```python
from build123d import *

# Parameters (mm, degrees)
SKETCH1_R                = 1.5
BOSS_EXTRUDE1_DEPTH      = 4
SKETCH2_W                = 10
SKETCH2_H                = 6
BOSS_EXTRUDE2_DEPTH      = 5
SKETCH7_W                = 6
SKETCH7_H                = 5
BOSS_EXTRUDE5_DEPTH      = 10
SKETCH4_R                = 2.5
BOSS_EXTRUDE3_DEPTH      = 10
BOSS_EXTRUDE3_DEPTH_BACK = 5


with BuildPart() as part:
    # Sketch1 → Boss-Extrude1 (new body)
    with BuildSketch(Plane.XY):
        Polygon((0, 0), (0, 30), (7.5, 30), (7.5, 0), (7.5, -2), (0, -2), align=None)
        with Locations((3.75, 26.5)):
            Circle(SKETCH1_R, mode=Mode.SUBTRACT)
        with Locations((3.75, 3.5)):
            Circle(SKETCH1_R, mode=Mode.SUBTRACT)
    extrude(amount=BOSS_EXTRUDE1_DEPTH)

    # Sketch2 → Boss-Extrude2 (add)
    with BuildSketch(Plane.XZ.offset(2)):
        with Locations((3.75, 3)):
            Rectangle(SKETCH2_W, SKETCH2_H)
    extrude(amount=BOSS_EXTRUDE2_DEPTH)

    # Sketch7 → Boss-Extrude5 (add)
    with BuildSketch(Plane.ZY.offset(1.25)):
        with Locations((3, -4.5)):
            Rectangle(SKETCH7_W, SKETCH7_H)
    extrude(amount=BOSS_EXTRUDE5_DEPTH)

    # Sketch4 → Boss-Extrude3 (add, two sides)
    with BuildSketch(Plane.XZ.offset(7)) as boss_extrude3_sk:
        with Locations((8.75, 3.5)):
            Circle(SKETCH4_R)
        with Locations((-11.25, 1.044308782)):
            Circle(SKETCH4_R)
    extrude(amount=BOSS_EXTRUDE3_DEPTH)
    extrude(boss_extrude3_sk.sketch, amount=-BOSS_EXTRUDE3_DEPTH_BACK)


solid = part.part
```
Could you check a few things on this model? Use its own coordinates, in mm. A direction names the side the tool comes from. Give positions to 0.01 mm unless a question says otherwise; leave off trailing zeros. Write each loop counter-clockwise with the first axis right and the second up, starting at its lowest first coordinate (ties: lowest second). Pieces come first, ordered by that corner, then holes. Notation, with made-up numbers: (34.25, 32.5) -> (57.25, 32.5) arc R22 ccw to (57.25, 69.5) -> close; hole circle Ø5 at (49.5, 2.5). An arc over 180 degrees is marked (long way). Write each question's results on one line, items separated by ' | '.
1. I want a section at B-B, the plane x = 3.75. Write out the boundary of the cut face in (y, z), then the cut area to 3 significant figures.
Check sheet entries:
outline: (-7, 0) -> (2, 0) -> (2, 4) -> (-2, 4) -> (-2, 6) -> (-7, 6) -> close; (5, 0) -> (25, 0) -> (25, 4) -> (5, 4) -> close; (28, 0) -> (30, 0) -> (30, 4) -> (28, 4) -> close | area: 134 mm²
2. I want a section at D-D, the plane x = -7.75. Write out the boundary of the cut face in (y, z).
Check sheet entries:
outline: (-7, 0) -> (-2, 0) -> (-2, 6) -> (-7, 6) -> close
3. If we mould it in two halves opening along X, with no side actions, what happens to faces 1 (the cylindrical face through (5.136, 2.925, 1.972)), 2 (the flat face through (9, -17, 4)), 3 (the flat face through (8.75, -4.5, 0.5))? For each: released by +X, released by -X, zero draft, split by the parting line, or undercut.
Check sheet entries:
face 1: undercut | face 2: zero draft | face 3: released by +X
4. On a 3-axis mill with a long thin cutter (end or side, diameter ignored), from which of +Z, -Z, +X, -X, +Y, -Y can I reach the whole of each face in a straight line? I mean faces 4 (the flat face through (0, 14, 2)), 5 (the flat face through (7.5, 14, 2)), 6 (the flat face through (2, 7, 0)), 7 (the flat face through (4, 14, 4)). Say none if no direction works.
Check sheet entries:
face 4: +Z, -Z, -X, +Y | face 5: +Z, -Z, +X, +Y | face 6: -Z, +X, +Y, -Y | face 7: +Z, +X, -X, +Y
5. Will these pins go through, and if not, where does the flat tip stop? pin 1 Ø3 at (x, z) = (-0.5, 4.5) entering from -Y; pin 2 Ø4 at (x, y) = (8, -3.5) entering from -Z; pin 3 Ø3 at (x, z) = (-9.5, 1.5) entering from +Y.
Check sheet entries:
pin 1: stops at y = -7 | pin 2: stops at z = 0 | pin 3: stops at y = -2
6. I want a section at A-A, the plane y = 3.5. Write out the boundary of the cut face in (x, z), then the cut area to 3 significant figures.
Check sheet entries:
outline: (0, 0) -> (2.25, 0) -> (2.25, 4) -> (0, 4) -> close; (5.25, 0) -> (7.5, 0) -> (7.5, 4) -> (5.25, 4) -> close | area: 18.0 mm²
7. I want a section at C-C, the plane z = 4.5. Write out the boundary of the cut face in (x, y).
Check sheet entries:
outline: (-11.25, -7) -> (6.46, -7) -> (6.46, -17) -> (11.04, -17) -> (11.04, -2) -> (-11.25, -2) -> close
8. I need wall thicknesses on L1, parallel to Y at x = 3.75, z = 2.85; L2, parallel to Y at x = -7.25, z = 2; L3, parallel to Z at x = -3, y = -3. Which ranges of each line are inside material? Lowest first, please.
Check sheet entries:
L1: y = -7 to 2, 5 to 25, 28 to 30 | L2: y = -7 to -2 | L3: z = 0 to 6
